from build123d import *

# Parameters (mm, degrees)
F1_DEPTH = 2
F2_R     = 1
F3_DEPTH = 2.001
F4_R     = 8
F5_DEPTH = 3.5
F6_R     = 7
F7_DEPTH = 2
F8_R     = 2.5
F9_DEPTH = 2


with BuildPart() as f1:
    # F0 (on Top) → F1 (new body)
    with BuildSketch(Plane.XY):
        with BuildLine():
            Line((16.75, -33), (16.75, 33))
            ThreePointArc((16.75, 33), (11.844039, 44.844039), (0, 49.75))
            ThreePointArc((0, 49.75), (-11.844039, 44.844039), (-16.75, 33))
            Line((-16.75, 33), (-16.75, -33))
            ThreePointArc((-16.75, -33), (-11.844039, -44.844039), (0, -49.75))
            ThreePointArc((0, -49.75), (11.844039, -44.844039), (16.75, -33))
        make_face()
    extrude(amount=F1_DEPTH)

    # F2 (on face) → F3 (cut, through all)
    with BuildSketch(Plane.XY.offset(2)):
        with Locations((-13, -37.25)):
            Circle(F2_R)
        with Locations((13, -37.25)):
            Circle(F2_R)
        with Locations((0, 1.25)):
            Circle(F2_R)
        with Locations((0, -19.75)):
            Circle(F2_R)
        with Locations((13, 37.25)):
            Circle(F2_R)
        with Locations((-13, 37.25)):
            Circle(F2_R)
    extrude(amount=-F3_DEPTH, mode=Mode.SUBTRACT)

    # F4 (on face) → F5 (join)
    with BuildSketch(Plane.XY.offset(2)):
        with Locations((0, 33.25)):
            Circle(F4_R)
    extrude(amount=F5_DEPTH)

    # F6 (on face) → F7 (join)
    with BuildSketch(Plane.XY.offset(5.5)):
        with Locations((0, 33.25)):
            Circle(F6_R)
    extrude(amount=F7_DEPTH)

    # F8 (on face) → F9 (join)
    with BuildSketch(Plane.XY.offset(2)):
        with Locations((0, -32.75)):
            Circle(F8_R)
    extrude(amount=F9_DEPTH)


solid = f1.part
Part model, mm, in its own coordinate system. A direction names the side the tool comes from. Round coordinates to 2 decimals unless told otherwise and drop trailing zeros. Write each loop counter-clockwise with the first axis right and the second up, starting at its lowest first coordinate (ties: lowest second). Pieces come first, ordered by that corner, then holes. Notation, with made-up numbers: M 2,86 L 30,86 A20 ccw 30,107 Z; hole C -8,32 d8. An arc over 180 degrees is marked long. Return JSON: item names as keys, results as strings. Group by question number.
(1) Which spindle directions (+Z, -Z, +X, -X, +Y, -Y) get a long thin tool onto all of the face, cutting with end or side? Do faces 5 (the face through (0, -33, 4)), 6 (the face through (-13.13, 38.24, 1.01)), 7 (the face through (-0.33, -30.27, 2.99)). Say none if no direction does.
(2) Two-plate mould, pull along Y, no slides. Class faces 1 (the face through (-0.217, -20.726, 1.014)), 2 (the face through (12.87, 38.24, 1.01)), 3 (the face through (-0.91, 40.19, 6.49)), 4 (the face through (0, 26, 5.5)): +Y half, -Y half, draft (parallel to the pull), parting line (faces both ways), or undercut.
(3) Drill centre lines: probe 1 along Y at (x, z) = (-13, 1.05); probe 2 along Z at (x, y) = (15, 24); probe 3 along Y at (x, z) = (-4.5, 3.75). Where is each one in solid material? Low to high.
(4) Pin check, flat tips, straight feed: pin 1 Ø17 at (x, y) = (-1, -16.5) entering from +Z; pin 2 Ø2.5 at (x, y) = (1, -32) entering from +Z. Stop position of each tip, or through.
(5) Saw through at A-A on y = -19.75. Write the cut outline in (x, z), then the cut area to 3 significant figures.
(6) Saw through at C-C on y = 37.25. Write the cut outline in (x, z).
(7) Saw through at B-B on x = 13. Write the cut outline in (y, z).
(8) Saw through at D-D on x = -5. Write the cut outline in (y, z) (3 decimals), then the cut area to 3 significant figures.
Returned:
{
 "1": {"face 5": "+Z, +X, -X, -Y", "face 6": "+Z, -Z", "face 7": "+Z"},
 "2": {"face 1": "undercut", "face 2": "undercut", "face 3": "parting line", "face 4": "draft"},
 "3": {"probe 1": "-43.56 to -38.25, -36.25 to 36.25, 38.25 to 43.56", "probe 2": "0 to 2", "probe 3": "26.64 to 39.86"},
 "4": {"pin 1": "z = 2", "pin 2": "z = 4"},
 "5": {"outline": "M -16.75,0 L -1,0 L -1,2 L -16.75,2 Z; M 1,0 L 16.75,0 L 16.75,2 L 1,2 Z", "area": "63.0 mm²"},
 "6": {"outline": "M -16.2,0 L -14,0 L -14,2 L -16.2,2 Z; M -12,0 L 12,0 L 12,2 L 6.93,2 L 6.93,5.5 L 5.74,5.5 L 5.74,7.5 L -5.74,7.5 L -5.74,5.5 L -6.93,5.5 L -6.93,2 L -12,2 Z; M 14,0 L 16.2,0 L 16.2,2 L 14,2 Z"},
 "7": {"outline": "M -43.56,0 L -38.25,0 L -38.25,2 L -43.56,2 Z; M -36.25,0 L 36.25,0 L 36.25,2 L -36.25,2 Z; M 38.25,0 L 43.56,0 L 43.56,2 L 38.25,2 Z"},
 "8": {"outline": "M -48.986,0 L 48.986,0 L 48.986,2 L 39.495,2 L 39.495,5.5 L 38.149,5.5 L 38.149,7.5 L 28.351,7.5 L 28.351,5.5 L 27.005,5.5 L 27.005,2 L -48.986,2 Z", "area": "259 mm²"}
}
